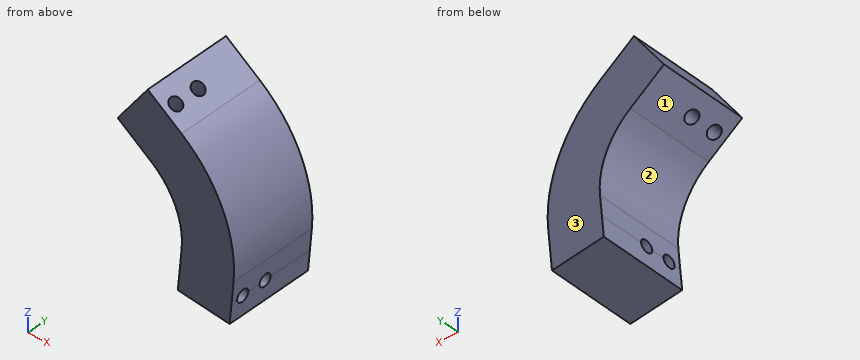
Autodesk Inventor part; units mm, degrees
ref_plane "YZ Plane" through (0, 0, 0) normal (1, 0, 0) x (0, 1, 0)
ref_plane "XZ Plane" through (0, 0, 0) normal (0, 1, 0) x (-1, 0, 0)
ref_plane "XY Plane" through (0, 0, 0) normal (0, 0, 1) x (1, 0, 0)
sketch "Sketch1" plane through (0, 0, 0) normal (0, 1, 0) x (-1, 0, 0)
  arc A0 (7.3141, 15.8982) -> (0, 0) centre (17.4253, 1.6149) ccw
  arc A1 (0.0437, 26.1686) -> (-12.541, -1.0355) centre (17.4253, 1.6149) ccw
  line L0 (7.3141, 15.8982) -> (0.0437, 26.1686)
  line L1 (7.3141, 15.8982) -> (15.476, 21.6761)
  line L2 (0.0437, 26.1686) -> (9.8323, 33.098)
  line L3 (15.476, 21.6761) -> (8.2056, 31.9464)
  line L4 (11.395, 18.7872) -> (4.1246, 29.0575)
  line L5 (0, 0) -> (0.4614, -4.9787)
  line L6 (0.4614, -4.9787) -> (-12.0679, -6.1398)
  line L7 (-12.0679, -6.1398) -> (-12.541, -1.0355)
  line L8 (0.4614, -4.9787) -> (0.9228, -9.9573)
  line L9 (0.9228, -9.9573) -> (-11.6065, -11.1185)
  line L10 (-12.0679, -6.1398) -> (-11.6065, -11.1185)
  dimension "d3" = 10
  dimension "d5" = 12.5833
  dimension "d6" = 12.5833
  dimension "d8" = 17.5
  dimension "d9" = 5
  dimension "d11" = 5
  dimension "d12" = 12.583
  dimension "d13" = 60
  dimension "d14" = 90
  dimension "d16" = 90
  dimension "d17" = 5
extrude "Extrusion1" add sketch "Sketch1" along normal blind 21
sketch "Sketch2" plane through (0, 0, 0) normal (-0.9957, 0, 0.0923) x (0.0923, 0, 0.9957)
  circle A0 centre (-5, 9) radius 1.5
  line L0 (-10, 0) -> (0, 0)
  circle A1 centre (-5, 3) radius 1.5
  line L1 (-10, 0) -> (-10, 21)
  dimension "d20" = 3
  dimension "d22" = 3
  dimension "d23" = 6
  dimension "d24" = 3
  dimension "d25" = 5
  dimension "d26" = 5
sketch "Sketch3" plane through (-15.476, 0, 21.6761) normal (-0.5778, 0, -0.8162) x (-0.8162, 0, 0.5778)
  circle A0 centre (-5, 3) radius 1.5
  circle A1 centre (-5, 9) radius 1.5
  line L0 (-10, 0) -> (0, 0)
  line L1 (0, 0) -> (0, 21)
  point P0 (-25.1554, 0)
  dimension "d27" = 3
  dimension "d28" = 3
  dimension "d29" = 6
  dimension "d30" = 0
  dimension "d31" = 3
  dimension "d32" = 5
extrude "Extrusion2" cut sketch "Sketch3" against normal blind 300
extrude "Extrusion3" cut sketch "Sketch2" against normal through all
properties part number "Soporte"
Work out the finished part from the listing and answer in its coordinate system (mm). Face numbers are marked on the shaded views. Give positions to 0.01 mm unless a question says otherwise; leave off trailing zeros. Loops run counter-clockwise (first coordinate to the right, second up) from the corner with the lowest first, then second, coordinate; pieces in that order, holes last. Notation, with made-up numbers: (12.25, -17.5) - (39.25, -17.5) arc R17 ccw to (39.25, 5.5) - close; hole circle Ø7 at (49, -33). An arc over 180 degrees is marked (long way). Answer in a Markdown table with one row per item.
(1) Section A-A (y = 8.25) is taken. Give the vertices of the cut face in (x, z).
Results list:
| item | result |
|---|---|
| outline | (-15.48, 21.68) - (-12.46, 19.54) - (-5.18, 29.81) - (-8.21, 31.95) - close; (-10.33, 18.04) - (-7.31, 15.9) arc R17.5 cw to (0, 0) - (-0.34, -3.69) - (12.19, -4.85) - (12.54, -1.04) arc R30.08 ccw to (-0.04, 26.17) - (-3.06, 28.31) - close; (-0.92, -9.96) - (11.61, -11.12) - (11.95, -7.43) - (-0.58, -6.27) - close |
(2) Flat-ended cylindrical pins translate along their axes: pin 1 Ø1 at (x, y) = (-2, 17.5) entering from -Z; pin 2 Ø1 at (y, z) = (9.5, 14.5) entering from +X; pin 3 Ø1.5 at (x, y) = (6, 17.5) entering from +Z. Find the tip coordinate at first contact, or state that the pin passes through.
Results list:
| item | result |
|---|---|
| pin 1 | stops at z = 8.87 |
| pin 2 | stops at x = 9.99 |
| pin 3 | stops at z = 21.38 |
(3) Consider L1, parallel to X at y = 1.75, z = 24.5; L2, parallel to X at y = 7.75, z = 28; L3, parallel to X at y = 13.5, z = 22. Determine where each line is inside the solid, lowest interval first. Write a range as [from, to].
Results list:
| item | result |
|---|---|
| L1 | x = [-13.48, -8.37], [-6.33, 2.1] |
| L2 | x = [-11, -5.89], [-3.86, -2.63] |
| L3 | x = [-15.25, 4.7] |
(4) Section C-C (z = 6) is taken. Give the vertices of the cut face in (x, y), and give its area (3 significant figures).
Results list:
| item | result |
|---|---|
| outline | (-0.48, 0) - (12.34, 0) - (12.34, 21) - (-0.48, 21) - close |
| area | 269 mm² |
(5) Section B-B (y = 12.5) is taken. Give the vertices of the cut face in (x, z), and give its area (3 significant figures).
Results list:
| item | result |
|---|---|
| outline | (-15.48, 21.68) - (-7.31, 15.9) arc R17.5 cw to (0, 0) - (-0.46, -4.98) - (-0.92, -9.96) - (11.61, -11.12) - (12.07, -6.14) - (12.54, -1.04) arc R30.08 ccw to (-0.04, 26.17) - (-8.21, 31.95) - close |
| area | 565 mm² |
(6) Section D-D (y = 4) is taken. Give the vertices of the cut face in (x, z).
Results list:
| item | result |
|---|---|
| outline | (-15.48, 21.68) - (-12.31, 19.43) - (-5.04, 29.7) - (-8.21, 31.95) - close; (-10.48, 18.14) - (-7.31, 15.9) arc R17.5 cw to (0, 0) - (-0.36, -3.87) - (12.17, -5.03) - (12.54, -1.04) arc R30.08 ccw to (-0.04, 26.17) - (-3.21, 28.41) - close; (-0.92, -9.96) - (11.61, -11.12) - (11.96, -7.25) - (-0.56, -6.09) - close |
(7) For a pull along Z with two mould halves and no side action, classify the marked faces 1, 2 and 3 as pulls with the +Z half, pulls with the -Z half, needs draft (parallel to the pull), parting line crosses it, or undercut.
Results list:
| item | result |
|---|---|
| face 1 | pulls with the -Z half |
| face 2 | undercut |
| face 3 | needs draft |
